from build123d import *

# Parameters (mm, degrees)
BOSS_EXTRUDE1_DEPTH     = 6.35
F_1_4_20_TAPPED_HOLE1_D = 5.1054
LPATTERN1_COUNT         = 4
LPATTERN1_PITCH         = 19.05


with BuildPart() as part:
    # Sketch1 → Boss-Extrude1 (new body)
    with BuildSketch(Plane(origin=(0, 0, 0), x_dir=(1, 0, 0), z_dir=(0, 1, 0))):
        with BuildLine():
            Line((-74.82695853, -9.525), (-15.875, -9.525))
            ThreePointArc((-15.875, -9.525), (-11.384871939, -11.384871939), (-9.525, -15.875))
            Line((-9.525, -15.875), (-9.525, -28.575))
            Line((-9.525, -28.575), (9.525, -28.575))
            Line((9.525, -28.575), (9.525, -15.875))
            ThreePointArc((9.525, -15.875), (11.384871939, -11.384871939), (15.875, -9.525))
            Line((15.875, -9.525), (45.485511374, -9.525))
            Line((45.485511374, -9.525), (45.485511374, 9.525))
            Line((45.485511374, 9.525), (15.875, 9.525))
            ThreePointArc((15.875, 9.525), (11.384871939, 11.384871939), (9.525, 15.875))
            Line((9.525, 15.875), (9.525, 28.575))
            Line((9.525, 28.575), (-9.525, 28.575))
            Line((-9.525, 28.575), (-9.525, 15.875))
            ThreePointArc((-9.525, 15.875), (-11.384871939, 11.384871939), (-15.875, 9.525))
            Line((-15.875, 9.525), (-75.059577466, 9.525))
            Line((-75.059577466, 9.525), (-82.55, 9.525))
            Line((-82.55, 9.525), (-82.55, -9.525))
            Line((-82.55, -9.525), (-74.82695853, -9.525))
        make_face()
    extrude(amount=BOSS_EXTRUDE1_DEPTH)

    # 1/4-20 Tapped Hole1 (through all)
    with Locations(Plane(origin=(0, 0, 0), x_dir=(-1, 0, 0), z_dir=(0, -1, 0))):
        with Locations((28.575, 0)):
            f_1_4_20_tapped_hole1 = Hole(F_1_4_20_TAPPED_HOLE1_D / 2)

    # LPattern1: 1/4-20 Tapped Hole1 ×4
    with Locations(*[(i * LPATTERN1_PITCH, 0, 0) for i in range(1, LPATTERN1_COUNT)]):
        add(f_1_4_20_tapped_hole1, mode=Mode.SUBTRACT)


solid = part.part
CAD build for the part. Positions are in the model's coordinates, mm. A direction names the side the tool comes from. Give positions to 0.01 mm unless a question says otherwise; leave off trailing zeros. Write each loop counter-clockwise with the first axis right and the second up, starting at its lowest first coordinate (ties: lowest second). Pieces come first, ordered by that corner, then holes. Notation, with made-up numbers: (-31.5, 76) -> (4.5, 76) arc R11 cw to (4.5, 87) -> close; hole circle Ø1 at (34, 46). An arc over 180 degrees is marked (long way). Return JSON: item names as keys, results as strings.
Item 1: Drill centre lines: probe 1 along X at (y, z) = (4.25, 1); probe 2 along Z at (x, y) = (-62, 0.5) (3 decimals); probe 3 along Z at (x, y) = (7.5, 2.25) (3 decimals). Where is each one in solid material? Low to high.
Answer below:
{"probe 1": "x = -82.55 to -30.92, -26.23 to -11.87, -7.18 to 7.18, 11.87 to 26.23, 30.92 to 45.49", "probe 2": "z = -9.525 to 9.525", "probe 3": "z = -28.575 to -1.554, 1.554 to 28.575"}
Item 2: Drop flat-ended pins along their axis: pin 1 (1.5 mm diameter, centred on y = 2.5, z = 18.5, fed in from -X) (3 decimals); pin 2 (2 mm diameter, centred on x = -21, y = 4, fed in from -Z) (3 decimals); pin 3 (1.9 mm diameter, centred on x = 33.5, y = 4.5, fed in from +Z) (3 decimals). Give the stop position or say it passes through.
Answer below:
{"pin 1": "stops at x = -9.525", "pin 2": "stops at z = -9.525", "pin 3": "stops at z = 9.525"}
Item 3: Band-saw the part on A-A (z = 0). List the corners of the cut face in (x, y).
Answer below:
{"outline": "(-82.55, 0) -> (-31.13, 0) -> (-31.13, 6.35) -> (-82.55, 6.35) -> close; (-26.02, 0) -> (-12.08, 0) -> (-12.08, 6.35) -> (-26.02, 6.35) -> close; (-6.97, 0) -> (6.97, 0) -> (6.97, 6.35) -> (-6.97, 6.35) -> close; (12.08, 0) -> (26.02, 0) -> (26.02, 6.35) -> (12.08, 6.35) -> close; (31.13, 0) -> (45.49, 0) -> (45.49, 6.35) -> (31.13, 6.35) -> close"}
Item 4: Two-plate mould, pull along X, no slides. Class faces 4 (the flat face through (-9.525, 3, -22)), 5 (the cylindrical face through (26.694, 3.219, -1.725)), 6 (the flat face through (9.525, 3, 22)): +X half, -X half, draft (parallel to the pull), parting line (faces both ways), or undercut.
Answer below:
{"face 4": "-X half", "face 5": "undercut", "face 6": "+X half"}
Item 5: Tool access for faces 1 (the flat face through (30, 3, 9.525)), 2 (the flat face through (-49, 3, -9.525)), 3 (the flat face through (31, 3, -9.525)): list every direction of +Z, -Z, +X, -X, +Y, -Y with a clear straight run to the whole face (end or side of a thin tool).
Answer below:
{"face 1": "+Z, +X, +Y, -Y", "face 2": "-Z, -X, +Y, -Y", "face 3": "-Z, +X, +Y, -Y"}
Item 6: Band-saw the part on B-B (y = 3). List the corners of the cut face in (x, z) (3 decimals).
Answer below:
{"outline": "(-82.55, -9.525) -> (-15.875, -9.525) arc R6.35 cw to (-9.525, -15.875) -> (-9.525, -28.575) -> (9.525, -28.575) -> (9.525, -15.875) arc R6.35 cw to (15.875, -9.525) -> (45.486, -9.525) -> (45.486, 9.525) -> (15.875, 9.525) arc R6.35 cw to (9.525, 15.875) -> (9.525, 28.575) -> (-9.525, 28.575) -> (-9.525, 15.875) arc R6.35 cw to (-15.875, 9.525) -> (-82.55, 9.525) -> close; hole circle Ø5.105 at (-28.575, 0); hole circle Ø5.105 at (-9.525, 0); hole circle Ø5.105 at (9.525, 0); hole circle Ø5.105 at (28.575, 0)"}
Item 7: Band-saw the part on C-C (x = -58). List the corners of the cut face in (y, z) (3 decimals).
Answer below:
{"outline": "(0, -9.525) -> (6.35, -9.525) -> (6.35, 9.525) -> (0, 9.525) -> close"}
Item 8: Band-saw the part on D-D (z = 19). List the corners of the cut face in (x, y) (3 decimals), then the cut area to 3 significant figures.
Answer below:
{"outline": "(-9.525, 0) -> (9.525, 0) -> (9.525, 6.35) -> (-9.525, 6.35) -> close", "area": "121 mm2"}
